Build history of the part. All positions in model axes, mm. A direction names the side the tool comes from. Coordinates: 2 decimals unless noted, no trailing zeros. Order: outer loops, then holes, each group sorted by start corner. A loop starts at its lowest first (then second) coordinate and runs counter-clockwise, first axis right, second up. Notation, with made-up numbers: (28.25, 25.25) - (33.25, 25.25) arc R16 cw to (33.25, 32.25) - close; hole circle Ø7 at (-21, 2.5). An arc over 180 degrees is marked (long way). Return JSON: item names as keys, results as strings.
from build123d import *

# Parameters (mm, degrees)
SKETCH_W     = 40
SKETCH_H     = 40
PAD_DEPTH    = 10
SKETCH003_R  = 12.5
POCKET_DEPTH = 6


with BuildPart() as part:
    # Sketch → Pad (new body)
    with BuildSketch(Plane.XY):
        Rectangle(SKETCH_W, SKETCH_H)
    extrude(amount=-PAD_DEPTH)

    # Sketch001 → Groove (revolve, cut)
    with BuildSketch(Plane.XZ):
        Polygon((0, 0), (0, -5), (2.5, -3.249481), (2.5, 0), align=None)
    revolve(axis=Axis((0, 0, 0), (0, 0, 1)), mode=Mode.SUBTRACT)

    # Sketch003 → Pocket (cut)
    with BuildSketch(Plane.XY):
        Circle(SKETCH003_R)
    extrude(amount=-POCKET_DEPTH, mode=Mode.SUBTRACT)


solid = part.part
1. Cut at B-B on z = -4.25. Give the cut face in (x, y), plus the area to 3 significant figures.
Check values:
{"outline": "(-20, -20) - (20, -20) - (20, 20) - (-20, 20) - close; hole circle Ø25 at (0, 0)", "area": "1,110 mm²"}
2. Mould opens along Y. For faces 1 (the flat face through (-20, 0, -5)), 2 (the cylindrical face through (11.923, 3.755, -2.958)), 3 (the flat face through (0, 20, -5)) say: pulls with the +Y half, pulls with the -Y half, needs draft (parallel to the pull), parting line crosses it, or undercut.
Check values:
{"face 1": "needs draft", "face 2": "undercut", "face 3": "pulls with the +Y half"}
3. Probe L1, parallel to Y at x = 0, z = -2.75; L2, parallel to X at y = 2, z = -2.5; L3, parallel to Z at x = 2, y = -12. List the from-to ranges inside material, lowest first.
Check values:
{"L1": "-20 to -12.5, 12.5 to 20", "L2": "-20 to -12.34, 12.34 to 20", "L3": "-10 to -6"}
4. Tool access for faces 4 (the flat face through (0, -20, -5)), 5 (the flat face through (0, 0, -6)): list every direction of +Z, -Z, +X, -X, +Y, -Y with a clear straight run to the whole face (end or side of a thin tool).
Check values:
{"face 4": "+Z, -Z, +X, -X, -Y", "face 5": "+Z"}
5. Cut at C-C on y = -3.5. Give the cut face in (x, z), plus the area to 3 significant figures.
Check values:
{"outline": "(-20, -10) - (20, -10) - (20, 0) - (12, 0) - (12, -6) - (-12, -6) - (-12, 0) - (-20, 0) - close", "area": "256 mm²"}
6. Drop flat-ended pins along their axis: pin 1 (1.5 mm diameter, centred on x = -14.5, y = 5, fed in from +Z); pin 2 (8 mm diameter, centred on x = -3.5, y = -2, fed in from +Z). Give the stop position or say it passes through.
Check values:
{"pin 1": "z = 0", "pin 2": "z = -6"}
7. Cut at A-A on x = -12. Give the cut face in (y, z), plus the area to 3 significant figures.
Check values:
{"outline": "(-20, -10) - (20, -10) - (20, 0) - (3.5, 0) - (3.5, -6) - (-3.5, -6) - (-3.5, 0) - (-20, 0) - close", "area": "358 mm²"}
